Source: CAD feature listing. Evaluate the final solid. Frame: model axes, mm. A direction names the side the tool comes from. Give positions to 0.01 mm unless a question says otherwise; leave off trailing zeros. Write each loop counter-clockwise with the first axis right and the second up, starting at its lowest first coordinate (ties: lowest second). Pieces come first, ordered by that corner, then holes. Notation, with made-up numbers: (11, 71.5) -> (56, 71.5) arc R28 ccw to (56, 103.5) -> close; hole circle Ø5 at (39, -20). An arc over 180 degrees is marked (long way). Use one line per item in the form item = value. Start each with the question number.
(1) Cut plane B-B, the plane y = 21. Output: boundary loops of the cut face in (x, z).
(2) First-contact query: P1, Ø2.5, axis at y = 4, z = 9, coming from the -X side; P2, Ø1.6, axis at x = 27, y = 26.5, coming from the +Z side; P3, Ø3.5, axis at y = 4, z = 25.5, coming from the +X side. Flat tips, straight axial feed; report the tip coordinate or a pass-through.
(3) Cut plane A-A, the plane z = 46.5. Output: boundary loops of the cut face in (x, y) (3 decimals).
(4) Material intervals for line 1 along X through (y, z) = (-26, 61); line 2 along Z through (x, y) = (-18.5, 24); line 3 along X through (y, z) = (1, 12), sorted ascending. Write a range as from..to.
(5) Set-up query: faces 1 (the face through (-22.99, -14.01, 53.93)), 2 (the face through (23.22, -14.24, 53.93)), 3 (the face through (-27, 27, 57.15)), 4 (the face through (14.01, -22.99, 53.93)). Return all of +Z, -Z, +X, -X, +Y, -Y with unobstructed straight access to the full face (end or side cutting, diameter ignored); none if empty.
(6) Draft query along Y for faces 5 (the face through (-7.559, -5.796, 0.711)), 6 (the face through (4, -5.601, 7)), 7 (the face through (0.083, 15.875, 53.931)). Return one class per face: pulls with the +Y half, pulls with the -Y half, needs draft (parallel to the pull), parting line crosses it, or undercut.
from build123d import *

# Parameters (mm, degrees)
F0_R     = 9.525
F1_DEPTH = 50.8
F2_R     = 9.525
F2_R_2   = 3.175
F3_DEPTH = 6.35
F4_DEPTH = 25.4
F6_DEPTH = 101.6
F5_R     = 12.7
F5_R_2   = 11.1125
F7_DEPTH = 19.05
F8_R     = 1.5875
F9_DEPTH = 19.05


with BuildPart() as f1:
    # F0 (on Top) → F1 (new body, symmetric)
    with BuildSketch(Plane.XY):
        Circle(F0_R)
    extrude(amount=F1_DEPTH, both=True)

    # F2 (on face) → F3 (join)
    with BuildSketch(Plane.XY.offset(50.8)):
        with BuildLine():
            ThreePointArc((14.7783039193, -5.7980477982), (15.5984165818, -2.9504279589), (15.875, 0))
            ThreePointArc((15.875, 0), (15.5984165818, 2.9504279589), (14.7783039193, 5.7980477982))
            ThreePointArc((14.7783039193, 5.7980477982), (11.2253201513, 11.2253201513), (5.7980477982, 14.7783039193))
            ThreePointArc((5.7980477982, 14.7783039193), (0, 15.875), (-5.7980477982, 14.7783039193))
            ThreePointArc((-5.7980477982, 14.7783039193), (-11.2253201513, 11.2253201513), (-14.7783039193, 5.7980477982))
            ThreePointArc((-14.7783039193, 5.7980477982), (-15.875, 0), (-14.7783039193, -5.7980477982))
            ThreePointArc((-14.7783039193, -5.7980477982), (-11.2253201513, -11.2253201513), (-5.7980477982, -14.7783039193))
            ThreePointArc((-5.7980477982, -14.7783039193), (0, -15.875), (5.7980477982, -14.7783039193))
            ThreePointArc((5.7980477982, -14.7783039193), (11.2253201513, -11.2253201513), (14.7783039193, -5.7980477982))
        make_face()
        Circle(F2_R, mode=Mode.SUBTRACT)
        with BuildLine():
            ThreePointArc((5.7980477982, 14.7783039193), (11.2253201513, 11.2253201513), (14.7783039193, 5.7980477982))
            Line((14.7783039193, 5.7980477982), (31.4308964237, 22.4506403027))
            ThreePointArc((31.4308964237, 22.4506403027), (31.4308964237, 31.4308964237), (22.4506403027, 31.4308964237))
            Line((22.4506403027, 31.4308964237), (5.7980477982, 14.7783039193))
        make_face()
        with Locations((26.9407683632, 26.9407683632)):
            Circle(F2_R_2, mode=Mode.SUBTRACT)
        with BuildLine():
            Line((-22.4506403027, -31.4308964237), (-5.7980477982, -14.7783039193))
            ThreePointArc((-5.7980477982, -14.7783039193), (-11.2253201513, -11.2253201513), (-14.7783039193, -5.7980477982))
            Line((-14.7783039193, -5.7980477982), (-31.4308964237, -22.4506403027))
            ThreePointArc((-31.4308964237, -22.4506403027), (-31.4308964237, -31.4308964237), (-22.4506403027, -31.4308964237))
        make_face()
        with Locations((-26.9407683632, -26.9407683632)):
            Circle(F2_R_2, mode=Mode.SUBTRACT)
        with BuildLine():
            Line((31.4308964237, -22.4506403027), (14.7783039193, -5.7980477982))
            ThreePointArc((14.7783039193, -5.7980477982), (11.2253201513, -11.2253201513), (5.7980477982, -14.7783039193))
            Line((5.7980477982, -14.7783039193), (22.4506403027, -31.4308964237))
            ThreePointArc((22.4506403027, -31.4308964237), (31.4308964237, -31.4308964237), (31.4308964237, -22.4506403027))
        make_face()
        with Locations((26.9407683632, -26.9407683632)):
            Circle(F2_R_2, mode=Mode.SUBTRACT)
        with BuildLine():
            ThreePointArc((-14.7783039193, 5.7980477982), (-11.2253201513, 11.2253201513), (-5.7980477982, 14.7783039193))
            Line((-5.7980477982, 14.7783039193), (-22.4506403027, 31.4308964237))
            ThreePointArc((-22.4506403027, 31.4308964237), (-31.4308964237, 31.4308964237), (-31.4308964237, 22.4506403027))
            Line((-31.4308964237, 22.4506403027), (-14.7783039193, 5.7980477982))
        make_face()
        with Locations((-26.9407683632, 26.9407683632)):
            Circle(F2_R_2, mode=Mode.SUBTRACT)
        Circle(F2_R)
    extrude(amount=F3_DEPTH)

    # F2 (on face) → F4 (join)
    with BuildSketch(Plane.XY.offset(50.8)):
        with Locations((-26.9407683632, 26.9407683632)):
            Circle(F2_R_2)
        with Locations((26.9407683632, 26.9407683632)):
            Circle(F2_R_2)
        with Locations((26.9407683632, -26.9407683632)):
            Circle(F2_R_2)
        with Locations((-26.9407683632, -26.9407683632)):
            Circle(F2_R_2)
    extrude(amount=F4_DEPTH)

    # F5 (on face) → F6 (cut)
    with BuildSketch(Plane.XY.offset(57.15)):
        Polygon((-5.6006181585, 2.2830683253), (-7.62, 0), (-5.6006181585, -2.2830683253), (-5.6006181585, -5.6006181585), (-2.2830683253, -5.6006181585), (0, -7.62), (2.2830683253, -5.6006181585), (5.6006181585, -5.6006181585), (5.6006181585, -2.2830683253), (7.62, 0), (5.6006181585, 2.2830683253), (5.6006181585, 5.6006181585), (2.2830683253, 5.6006181585), (0, 7.62), (-2.2830683253, 5.6006181585), (-5.6006181585, 5.6006181585), align=None)
    extrude(amount=-F6_DEPTH, mode=Mode.SUBTRACT)

    # F5 (on face) → F7 (join)
    with BuildSketch(Plane.XY.offset(57.15)):
        Circle(F5_R)
        Circle(F5_R_2, mode=Mode.SUBTRACT)
    extrude(amount=F7_DEPTH)

    # F8 (on face) → F9 (cut)
    with BuildSketch(Plane.XY.offset(76.2)):
        with Locations((26.9407683632, -26.9407683632)):
            Circle(F8_R)
        with Locations((-26.9407683632, -26.9407683632)):
            Circle(F8_R)
        with Locations((26.9407683632, 26.9407683632)):
            Circle(F8_R)
        with Locations((-26.9407683632, 26.9407683632)):
            Circle(F8_R)
    extrude(amount=-F9_DEPTH, mode=Mode.SUBTRACT)


solid = f1.part
Geometry says:
q1.outline = (-29.98, 50.8) -> (-12.02, 50.8) -> (-12.02, 57.15) -> (-29.98, 57.15) -> close; (12.02, 50.8) -> (29.98, 50.8) -> (29.98, 57.15) -> (12.02, 57.15) -> close
q2.P1 = -9.12
q2.P2 = 57.15
q2.P3 = 9.26
q3.outline = circle Ø19.05 at (0, 0); hole (-7.62, 0) -> (-5.601, -2.283) -> (-5.601, -5.601) -> (-2.283, -5.601) -> (0, -7.62) -> (2.283, -5.601) -> (5.601, -5.601) -> (5.601, -2.283) -> (7.62, 0) -> (5.601, 2.283) -> (5.601, 5.601) -> (2.283, 5.601) -> (0, 7.62) -> (-2.283, 5.601) -> (-5.601, 5.601) -> (-5.601, 2.283) -> close
q4.line_1 = -29.97..-28.22, -25.66..-23.91, 23.91..25.66, 28.22..29.97
q4.line_2 = 50.8..57.15
q4.line_3 = -9.47..-6.74, 6.74..9.47
q5.face_1 = +Z, -Z, -X
q5.face_2 = +Z, -Z, +X
q5.face_3 = +Z
q5.face_4 = +Z, -Z, -Y
q6.face_5 = parting line crosses it
q6.face_6 = undercut
q6.face_7 = pulls with the +Y half
